from build123d import *

# Parameters (mm, degrees)
SKETCH_1_W               = 58
SKETCH_1_H               = 46
EXTRUDE_509_DEPTH        = 12.5
SKETCH_3_W               = 36
SKETCH_3_H               = 46
CUT_EXTRUDE_752_DEPTH    = 40.067249711
SKETCH_11_R              = 1.75
CUT_EXTRUDE_1006_DEPTH   = 8
CUT_EXTRUDE_1504_DEPTH   = 9
CUT_EXTRUDE_1848_REACH   = 65.634
SKETCH_4_R               = 4.2
SKETCH_6_R               = 4
CUT_EXTRUDE_1985_DEPTH   = 11
SKETCH_7_W               = 6.25
SKETCH_7_H               = 20.5
CUT_EXTRUDE_2184_DEPTH   = 11
SKETCH_8_R               = 5.25
CUT_EXTRUDE_2361_DEPTH   = 2.25
SKETCH_9_R               = 1.1
CUT_EXTRUDE_2719_DEPTH   = 5.25
CUT_EXTRUDE_3116_DEPTH   = 40.067249711
CHAMFER_1_SIZE           = 1
FILLET_1_R               = 1
CUT_EXTRUDE_START        = -4
CUT_EXTRUDE_6414_DEPTH   = 1.4
CUT_EXTRUDE_6952_REACH   = 65.634
SKETCH_18_W              = 6
SKETCH_18_H              = 2.8
MIRROR_START             = -4
MIRROR_2_COPY_1_DEPTH    = 1.4
MIRROR_2_COPY_2_REACH    = 65.634
MIRROR_2_COPY_2_SKETCH_W = 6
MIRROR_2_COPY_2_SKETCH_H = 2.8


with BuildPart() as part:
    # Эскиз1 → Extrude 509 (new body)
    with BuildSketch(Plane.XY):
        Rectangle(SKETCH_1_W, SKETCH_1_H)
    extrude(amount=EXTRUDE_509_DEPTH)

    # Эскиз3 → Cut-Extrude 752 (cut, through all)
    with BuildSketch(Plane.XY.offset(12.5)):
        with Locations((0, 3)):
            Rectangle(SKETCH_3_W, SKETCH_3_H)
    extrude(amount=-CUT_EXTRUDE_752_DEPTH, mode=Mode.SUBTRACT)

    # Эскиз11 → Cut-Extrude 1006 (cut)
    with BuildSketch(Plane.XZ.offset(23)):
        with Locations(Location((-25, 5, 0), (0, 0, 270))):
            Circle(SKETCH_11_R)
        with Locations(Location((25, 5, 0), (0, 0, 270))):
            Circle(SKETCH_11_R)
    cut_extrude_1006 = extrude(amount=-CUT_EXTRUDE_1006_DEPTH, mode=Mode.SUBTRACT)

    # Mirror 1050: Cut-Extrude 1006 across plane
    add(cut_extrude_1006.mirror(Plane.ZX), mode=Mode.SUBTRACT)

    # Эскиз5 → Cut-Extrude 1504 (cut)
    with BuildSketch(Plane(origin=(29, 0, 0), x_dir=(0, 0, -1), z_dir=(1, 0, 0))):
        with BuildLine():
            Line((-9.688386067, 0.588050321), (-8.743490646, -12.48028976))
            ThreePointArc((-8.743490646, -12.48028976), (-6.25, -14.8), (-3.756509354, -12.48028976))
            Line((-3.756509354, -12.48028976), (-2.811613933, 0.588050321))
            ThreePointArc((-2.811613933, 0.588050321), (-6.25, 7.2), (-9.688386067, 0.588050321))
        make_face()
    extrude(amount=-CUT_EXTRUDE_1504_DEPTH, mode=Mode.SUBTRACT)

    # Эскиз4 → Cut-Extrude 1848 (cut, up to next)
    with BuildSketch(Plane(origin=(29, 0, 0), x_dir=(0, 0, -1), z_dir=(1, 0, 0)), mode=Mode.PRIVATE) as cut_extrude_1848_sk1:
        with Locations((-6.25, 3)):
            Circle(SKETCH_4_R)
    cut_extrude_1848_tool1 = extrude(cut_extrude_1848_sk1.sketch, amount=-CUT_EXTRUDE_1848_REACH, mode=Mode.PRIVATE) & part.part
    add(cut_extrude_1848_tool1.solids().sort_by_distance((29, 3, 6.25))[0], mode=Mode.SUBTRACT)

    # Эскиз6 → Cut-Extrude 1985 (cut)
    with BuildSketch(Plane.ZY.offset(29)):
        with Locations((6.25, 3)):
            Circle(SKETCH_6_R)
    extrude(amount=-CUT_EXTRUDE_1985_DEPTH, mode=Mode.SUBTRACT)

    # Эскиз7 → Cut-Extrude 2184 (cut)
    with BuildSketch(Plane.ZY.offset(29)):
        with Locations((9.375, 3)):
            Rectangle(SKETCH_7_W, SKETCH_7_H)
    extrude(amount=-CUT_EXTRUDE_2184_DEPTH, mode=Mode.SUBTRACT)

    # Эскиз8 → Cut-Extrude 2361 (cut, symmetric)
    with BuildSketch(Plane.ZY.offset(23.5)):
        with Locations((6.25, 3)):
            Circle(SKETCH_8_R)
    extrude(amount=CUT_EXTRUDE_2361_DEPTH, both=True, mode=Mode.SUBTRACT)

    # Эскиз9 → Cut-Extrude 2719 (cut)
    with BuildSketch(Plane.XY.offset(6.25)):
        with Locations((-23.5, 10)):
            Circle(SKETCH_9_R)
        with Locations((-23.5, -4)):
            Circle(SKETCH_9_R)
    extrude(amount=-CUT_EXTRUDE_2719_DEPTH, mode=Mode.SUBTRACT)

    # Эскиз10 → Cut-Extrude 3116 (cut, through all)
    with BuildSketch(Plane.XY.offset(12.5)):
        Polygon((29, -13.165806523), (29, 9.565806523), (22.5, 7.2), (22.5, -10.8), align=None)
    extrude(amount=-CUT_EXTRUDE_3116_DEPTH, mode=Mode.SUBTRACT)

    # Фаска1
    chamfer_1_edges = [part.edges().sort_by_distance(p)[0] for p in [
        (-29, 3, 2.25),
        (-18, 3, 2.25),
    ]]
    chamfer(chamfer_1_edges, length=CHAMFER_1_SIZE)

    # Скругление1
    fillet_1_edges = [part.edges().sort_by_distance(p)[0] for p in [
        (-18, -20, 6.25),
        (18, -20, 6.25),
    ]]
    fillet(fillet_1_edges, radius=FILLET_1_R)

    # Эскиз17 → Cut-Extrude 6414 (cut, symmetric)
    with BuildSketch(Plane(origin=(0, 23, 0), x_dir=(1, 0, 0), z_dir=(0, 1, 0)).offset(CUT_EXTRUDE_START)):
        Polygon((22, -3.267949192), (22, -6.732050808), (25, -8.464101615), (28, -6.732050808), (28, -3.267949192), (25, -1.535898385), align=None)
    cut_extrude_6414 = extrude(amount=CUT_EXTRUDE_6414_DEPTH, both=True, mode=Mode.SUBTRACT)

    # Эскиз18 → Cut-Extrude 6952 (cut, up to next)
    with BuildSketch(Plane(origin=(29, 0, 12.5), x_dir=(1, 0, 0), z_dir=(0, 0, 1)), mode=Mode.PRIVATE) as cut_extrude_6952_sk1:
        with Locations((-4, 19)):
            Rectangle(SKETCH_18_W, SKETCH_18_H)
    cut_extrude_6952_tool1 = extrude(cut_extrude_6952_sk1.sketch, amount=-CUT_EXTRUDE_6952_REACH, mode=Mode.PRIVATE) & part.part
    cut_extrude_6952 = cut_extrude_6952_tool1.solids().sort_by_distance((25, 19, 12.5))[0]
    add(cut_extrude_6952, mode=Mode.SUBTRACT)

    # Зеркальное отражение1: Cut-Extrude 6414, Cut-Extrude 6952 across plane
    add(cut_extrude_6414.mirror(Plane(origin=(0, 0, 0), x_dir=(0, 0, 1), z_dir=(1, 0, 0))), mode=Mode.SUBTRACT)
    add(cut_extrude_6952.mirror(Plane(origin=(0, 0, 0), x_dir=(0, 0, 1), z_dir=(1, 0, 0))), mode=Mode.SUBTRACT)

    # Зеркальное отражение2: Cut-Extrude 6414, Cut-Extrude 6952 across plane
    add(cut_extrude_6414.mirror(Plane.ZX), mode=Mode.SUBTRACT)
    add(cut_extrude_6952.mirror(Plane.ZX), mode=Mode.SUBTRACT)

    # Зеркальное отражение2 copy 1 sketch → Зеркальное отражение2 copy 1 (cut, symmetric)
    with BuildSketch(Plane(origin=(0, -23, 0), x_dir=(-1, 0, 0), z_dir=(0, -1, 0)).offset(MIRROR_START)):
        Polygon((22, -3.267949192), (22, -6.732050808), (25, -8.464101615), (28, -6.732050808), (28, -3.267949192), (25, -1.535898385), align=None)
    extrude(amount=MIRROR_2_COPY_1_DEPTH, both=True, mode=Mode.SUBTRACT)

    # Зеркальное отражение2 copy 2 sketch → Зеркальное отражение2 copy 2 (cut, up to next)
    with BuildSketch(Plane(origin=(-29, 0, 12.5), x_dir=(-1, 0, 0), z_dir=(0, 0, 1)), mode=Mode.PRIVATE) as mirror_2_copy_2_sk1:
        with Locations((-4, 19)):
            Rectangle(MIRROR_2_COPY_2_SKETCH_W, MIRROR_2_COPY_2_SKETCH_H)
    mirror_2_copy_2_tool1 = extrude(mirror_2_copy_2_sk1.sketch, amount=-MIRROR_2_COPY_2_REACH, mode=Mode.PRIVATE) & part.part
    add(mirror_2_copy_2_tool1.solids().sort_by_distance((-25, -19, 12.5))[0], mode=Mode.SUBTRACT)


solid = part.part
Work out the finished part from the listing and answer in its coordinate system (mm). A direction names the side the tool comes from. Give positions to 0.01 mm unless a question says otherwise; leave off trailing zeros. Loops run counter-clockwise (first coordinate to the right, second up) from the corner with the lowest first, then second, coordinate; pieces in that order, holes last. Notation, with made-up numbers: (27.5, 83.5) -> (86.5, 83.5) arc R23 ccw to (86.5, 101.5) -> close; hole circle Ø9 at (11.5, 87). An arc over 180 degrees is marked (long way). Use a Markdown table: item, result. Add a question column.
1. Section D-D on x = 13 is taken. Determine the outline of the cut face in (y, z).
2. Find the intervals of material crossed by probe 1 along X at (y, z) = (21.2, 5); probe 2 along X at (y, z) = (19.5, 4.5); probe 3 along X at (y, z) = (20.5, 7), in increasing order.
3. Section A-A on y = 3 is taken. Determine the outline of the cut face in (x, z), and give its area (3 significant figures).
4. For faces 1 (the flat face through (-21.25, 3, 2)), 2 (the flat face through (22.5, -2, 2)), 3 (the cylindrical face through (26.735, -16.318, 5.228)), 4 (the flat face through (21.236, -5.855, 9.223)), determine the directions among +Z, -Z, +X, -X, +Y, -Y from which every point of the face is accessible in a straight line to the end or side of a thin tool.
5. Section B-B on z = 5 is taken. State how many separate pieces and enclosed holes the cut face has, and give its area (3 significant figures).
6. Determine the mould class of faces 5 (the flat face through (-23.5, -19, 2.4)), 6 (the flat face through (-18, -3, 5)), 7 (the flat face through (25, -15, 5)), 8 (the flat face through (-25, 15, 5)) for opening direction Y: released by +Y, released by -Y, zero draft, split by the parting line, or undercut.
7. Section C-C on y = -4 is taken. Determine the outline of the cut face in (x, z), and give its area (3 significant figures).
8. Flat-ended cylindrical pins translate along their axes: pin 1 Ø0.7 at (x, y) = (-23, 10) entering from +Z; pin 2 Ø2.5 at (y, z) = (0.5, 3.5) entering from +X; pin 3 Ø3 at (x, z) = (-25, 5) entering from +Y; pin 4 Ø12 at (x, y) = (-8, -3) entering from +Z. Find the tip coordinate at first contact, or state that the pin passes through.
Results below:
| question | item | result |
|---|---|---|
| 1 | outline | (-23, 0) -> (-20, 0) -> (-20, 12.5) -> (-23, 12.5) -> close |
| 2 | probe 1 | x = -29 to -26.75, -23.25 to -18, 18 to 23.25, 26.75 to 29 |
| 2 | probe 2 | x = -29 to -28, -22 to -18, 18 to 22, 28 to 29 |
| 2 | probe 3 | x = -29 to -18, 18 to 29 |
| 3 | outline | (-29, 0) -> (-18, 0) -> (-18, 1.25) -> (-19, 2.25) -> (-21.25, 2.25) -> (-21.25, 1) -> (-25.75, 1) -> (-25.75, 2.25) -> (-28, 2.25) -> (-29, 1.25) -> close; (18, 0) -> (22.5, 0) -> (22.5, 2.05) -> (18, 2.05) -> close; (18, 10.45) -> (22.5, 10.45) -> (22.5, 12.5) -> (18, 12.5) -> close |
| 3 | area | 36.6 mm^2 |
| 4 | face 1 | +Z |
| 4 | face 2 | +Z, -Z, +X |
| 4 | face 3 | -Y |
| 4 | face 4 | +X |
| 5 | separate pieces | 3 |
| 5 | enclosed holes | 2 |
| 5 | area | 657 mm^2 |
| 6 | face 5 | undercut |
| 6 | face 6 | zero draft |
| 6 | face 7 | released by -Y |
| 6 | face 8 | released by +Y |
| 7 | outline | (-29, 0) -> (-18, 0) -> (-18, 6.25) -> (-22.4, 6.25) -> (-22.4, 1) -> (-24.6, 1) -> (-24.6, 6.25) -> (-29, 6.25) -> close; (18, 0) -> (22.5, 0) -> (22.5, 3.14) -> (20, 3.14) -> (20, 9.36) -> (22.5, 9.36) -> (22.5, 12.5) -> (18, 12.5) -> close |
| 7 | area | 97.9 mm^2 |
| 8 | pin 1 | stops at z = 1 |
| 8 | pin 2 | stops at x = 22.5 |
| 8 | pin 3 | stops at y = 15 |
| 8 | pin 4 | passes through |
